Autodesk Inventor part; units mm, degrees
ref_plane "Work Plane1" through (0, 3.175, 0) normal (0, -1, 0) x (1, 0, 0)
ref_plane "Work Plane2" through (0, 3.175, 17.145) normal (0.3003, 0, -0.9538) x (0, 1, 0)
ref_plane "YZ Plane" through (0, 0, 0) normal (1, 0, 0) x (0, 1, 0)
sketch "Sketch1" plane through (0, 0, 0) normal (0, 0, 1) x (1, 0, 0)
  line L0 (0, 3.175) -> (0, 0)
  line L1 (0, 0) -> (10.795, 0)
  line L2 (10.795, 0) -> (10.795, 6.831)
  arc A0 (0, 3.175) -> (10.795, 6.831) centre (-10.795, 52.8148) ccw
  line L3 (0, 3.175) -> (-10.795, 3.175) construction
  line L4 (-10.795, 3.175) -> (-10.795, 2.0148) construction
  arc A1 (-10.795, 2.0148) -> (0, 3.175) centre (-10.795, 52.8148) ccw construction
  dimension "d0" = 50.8
  dimension "d1" = 3.175
  dimension "d4" = 10.795
  dimension "d11" = 10.795
extrude "Extrusion1" add sketch "Sketch1" along normal blind 25.4
ref_plane "Work Plane1" through (0, 3.175, 0) normal (0, -1, 0) x (1, 0, 0)
sketch "Sketch2" plane through (0, 3.175, 0) normal (0, -1, 0) x (1, 0, 0)
  line L0 (0, 0) -> (0, 25.4)
  line L1 (0, 17.145) -> (5.3975, 0)
  line L2 (10.795, 0) -> (0, 0)
  line L3 (0, 25.4) -> (10.795, 25.4)
  dimension "d6" = 8.255
ref_plane "Work Plane2" through (0, 3.175, 17.145) normal (0.3003, 0, -0.9538) x (0, 1, 0)
sketch "Sketch3" plane through (0, 3.175, 17.145) normal (0.3003, 0, -0.9538) x (0, 1, 0)
  line L0 (2.2225, -1.905) -> (-2.2225, -1.905)
  line L1 (-2.2225, -1.905) -> (-2.2225, 1.905)
  line L2 (-2.2225, 1.905) -> (2.2225, 1.905)
  line L3 (2.2225, 1.905) -> (2.2225, -1.905)
  point P0 (-3.175, -5.1484)
  point P1 (0, 0)
  point P2 (2.2225, 0)
  point P3 (0, 1.905)
  dimension "d7" = 4.445
  dimension "d10" = 3.81
extrude "Extrusion2" cut sketch "Sketch3" along normal through all both and the other way through all
chamfer "Chamfer1" distance 2.54 angle 45 1 edges at (10.795, 0, 12.7)
chamfer "Chamfer2" distance 2.54 angle 45 1 edges at (4.1275, 0, 25.4)
properties part number "WireGuideToSail1" material "ABS Plastic"
Can you work these out from the model? Positions are in its coordinate system, mm. A direction names the side the tool comes from. Give positions to 0.01 mm unless a question says otherwise; leave off trailing zeros. Order: outer loops, then holes, each group sorted by start corner. A loop starts at its lowest first (then second) coordinate and runs counter-clockwise, first axis right, second up. Notation, with made-up numbers: M -30,22 L 27,22 A13 ccw 27,40 Z; hole C 61,79 d2. An arc over 180 degrees is marked long. One line per item, written item: value.
Item 1: If we section it at B-B on z = 5.75: Write out the boundary of the cut face in (x, y) (1 decimal).
Verdict:
outline: M 0,0 L 8.3,0 L 10.8,2.5 L 10.8,6.8 A50.8 cw 5.6,4.7 L 5.6,1 L 1.6,1 L 1.6,3.5 A50.8 cw 0,3.2 Z
Item 2: If we section it at C-C on y = 1.5: Write out the boundary of the cut face in (x, z) (3 decimals).
Verdict:
outline: M 0,0 L 3.401,0 L 0,10.802 Z; M 0,23.488 L 7.395,0 L 9.755,0 L 9.755,24.36 L 0,24.36 Z
Item 3: Please list where these lines run through material, in increasing order: line 1 (Y direction, x = 3.75, z = 6.25); line 2 (X direction, y = 1.25, z = 10) (3 decimals); line 3 (Y direction, x = 9.75, z = 23) (3 decimals).
Verdict:
line 1: 0 to 0.95
line 2: 0 to 0.252, 4.247 to 9.505
line 3: 1.495 to 6.355
Item 4: If we section it at D-D on x = 4.5: Write out the boundary of the cut face in (y, z).
Verdict:
outline: M 0,0 L 0.95,0 L 0.95,9.2 L 4.37,9.2 L 4.37,25.4 L 2.54,25.4 L 0,22.86 Z
Item 5: For pin 1 (3.5 mm diameter, centred on x = 4, z = 8, fed in from +Y), with a flat end and sliding along its axis, tell me the tip position at first contact or that it passes through.
Verdict:
pin 1: y = 4.78
Item 6: If we mould it in two halves opening along Z, with no side actions, what happens to faces 3 (the face through (0, 1, 10)), 4 (the face through (8, 3, 0)), 5 (the face through (3, 0.952, 9)), 6 (the face through (1.677, 2.174, 5.476))? For each: pulls with the +Z half, pulls with the -Z half, needs draft (parallel to the pull), parting line crosses it, or undercut.
Verdict:
face 3: needs draft
face 4: pulls with the -Z half
face 5: undercut
face 6: undercut
Item 7: If we section it at A-A on y = 3.75: Write out the boundary of the cut face in (x, z) (3 decimals).
Verdict:
outline: M 2.369,0 L 3.401,0 L 2.369,3.278 Z; M 2.369,15.964 L 7.395,0 L 10.795,0 L 10.795,25.4 L 2.369,25.4 Z
Item 8: For faces 1 (the face through (4.468, 2.645, 9.299)), 2 (the face through (0.974, 3.397, 2.925)), which set-ups out of +Z, -Z, +X, -X, +Y, -Y let a thin tool reach every point of the face, with its end or its side?
Verdict:
face 1: +Y
face 2: +Z, -Z, -X, +Y
